Autodesk Inventor part; units mm, degrees
ref_plane "YZ Plane" through (0, 0, 0) normal (1, 0, 0) x (0, 1, 0)
ref_plane "XY Plane" through (0, 0, 0) normal (0, 0, 1) x (1, 0, 0)
ref_plane "Work Plane1" through (0, 127, 0) normal (0, 1, 0) x (-1, 0, 0)
sketch "Sketch1" plane through (0, 127, 0) normal (0, 1, 0) x (-1, 0, 0)
  line L0 (0, 0) -> (25.4, 0)
  line L1 (25.4, 0) -> (25.4, -50.8)
  line L2 (25.4, -50.8) -> (0, -50.8)
  line L3 (0, -50.8) -> (0, 0)
  dimension "d1" = 25.4
  dimension "d2" = 50.8
extrude "Extrusion1" add sketch "Sketch1" along normal blind 25.4
fillet "Fillet1" radius 3.175 8 edges at (-12.7, 152.4, 0) (0, 139.7, 0) (0, 152.4, -25.4) (0, 139.7, -50.8) (-12.7, 152.4, -50.8) (0, 127, -25.4) (-12.7, 127, 0) (-12.7, 127, -50.8)
shell "Shell1" thickness 2.54 removed faces 0
sketch "Sketch2" plane through (0, 130.175, -47.625) normal (1, 0, 0) x (0, 0, -1)
  point P0 (-47.625, -130.175)
  point P1 (-33.1289, 9.839)
  point P2 (-11.4516, 9.7569)
hole "Hole1" at (0, 139.9319, -36.1734) at (0, 140.014, -14.4961) direction (-1, 0, 0) diameter 15.24 depth 2.54
properties part number "Ultrasonic Case"
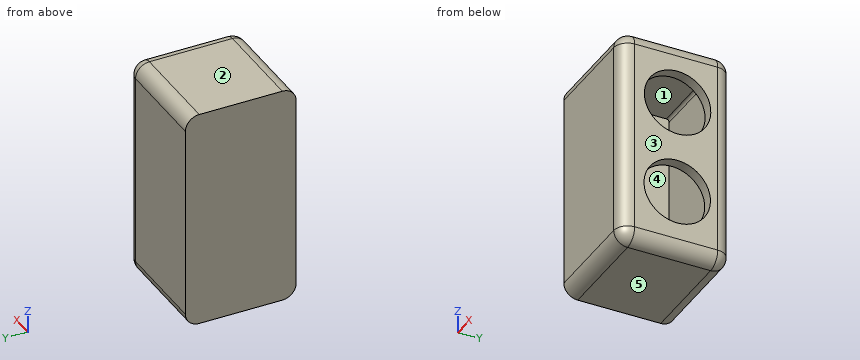
Build history of the part. All positions in model axes, mm. Face numbers are marked on the shaded views. A direction names the side the tool comes from. Round coordinates to 2 decimals unless told otherwise and drop trailing zeros. Loops run counter-clockwise (first coordinate to the right, second up) from the corner with the lowest first, then second, coordinate; pieces in that order, holes last. Notation, with made-up numbers: (60, -7.5) -> (91, -7.5) arc R36 cw to (91, 29.5) -> close; hole circle Ø4 at (48, 44.5). An arc over 180 degrees is marked (long way). Answer in a Markdown table with one row per item.
Item 1: Saw through at C-C (x = -11). Write the cut outline in (y, z) (3 decimals).
Answers below:
| item | result |
|---|---|
| outline | (127, -47.625) arc R3.175 ccw to (130.175, -50.8) -> (149.225, -50.8) arc R3.175 ccw to (152.4, -47.625) -> (152.4, -3.175) arc R3.175 ccw to (149.225, 0) -> (130.175, 0) arc R3.175 ccw to (127, -3.175) -> close; hole (129.54, -47.625) arc R0.635 ccw to (130.175, -48.26) -> (149.225, -48.26) arc R0.635 ccw to (149.86, -47.625) -> (149.86, -3.175) arc R0.635 ccw to (149.225, -2.54) -> (130.175, -2.54) arc R0.635 ccw to (129.54, -3.175) -> close |
Item 2: Saw through at A-A (y = 131.25). Write the cut outline in (x, z) (3 decimals), and give its area (3 significant figures).
Answers below:
| item | result |
|---|---|
| outline | (-25.4, -50.8) -> (-3.175, -50.8) arc R3.175 ccw to (0, -47.625) -> (0, -3.175) arc R3.175 ccw to (-3.175, 0) -> (-25.4, 0) -> close; hole (-22.86, -48.26) -> (-3.175, -48.26) arc R0.635 ccw to (-2.54, -47.625) -> (-2.54, -3.175) arc R0.635 ccw to (-3.175, -2.54) -> (-22.86, -2.54) -> close |
| area | 357 mm² |
Item 3: Mould opens along X. For the marked faces 3, 4 and 5 say: +X half, -X half, draft (parallel to the pull), parting line (faces both ways), or undercut.
Answers below:
| item | result |
|---|---|
| face 3 | +X half |
| face 4 | undercut |
| face 5 | draft |
Item 4: Saw through at B-B (z = -45.5). Write the cut outline in (x, y) (3 decimals).
Answers below:
| item | result |
|---|---|
| outline | (-25.4, 127) -> (-3.175, 127) arc R3.175 ccw to (0, 130.175) -> (0, 149.225) arc R3.175 ccw to (-3.175, 152.4) -> (-25.4, 152.4) -> close; hole (-22.86, 129.54) -> (-3.175, 129.54) arc R0.635 ccw to (-2.54, 130.175) -> (-2.54, 149.225) arc R0.635 ccw to (-3.175, 149.86) -> (-22.86, 149.86) -> close |
Item 5: Drill centre lines: L1, parallel to Y at x = -13.5, z = -23.5; L2, parallel to X at y = 148.5, z = -29.5; L3, parallel to Z at x = -18.25, y = 141.5. Where is each one in solid material? Low to high. Write a range as [from, to].
Answers below:
| item | result |
|---|---|
| L1 | y = [127, 129.54], [149.86, 152.4] |
| L2 | x = [-25.4, -22.86], [-2.54, 0] |
| L3 | z = [-50.8, -48.26], [-2.54, 0] |
Item 6: Which spindle directions (+Z, -Z, +X, -X, +Y, -Y) get a long thin tool onto all of the face, cutting with end or side? Do the marked faces 1 and 2. Say none if no direction does.
Answers below:
| item | result |
|---|---|
| face 1 | none |
| face 2 | +Z, +X, -X, +Y, -Y |
Item 7: Saw through at D-D (y = 134.5). Write the cut outline in (x, z) (3 decimals).
Answers below:
| item | result |
|---|---|
| outline | (-25.4, -50.8) -> (-3.175, -50.8) arc R3.175 ccw to (0, -47.625) -> (0, -41.517) -> (-2.54, -41.517) -> (-2.54, -47.625) arc R0.635 cw to (-3.175, -48.26) -> (-22.86, -48.26) -> (-22.86, -2.54) -> (-3.175, -2.54) arc R0.635 cw to (-2.54, -3.175) -> (-2.54, -9.237) -> (0, -9.237) -> (0, -3.175) arc R3.175 ccw to (-3.175, 0) -> (-25.4, 0) -> close; (-2.54, -30.829) -> (0, -30.829) -> (0, -19.755) -> (-2.54, -19.755) -> close |
